from build123d import *

# Parameters (mm, degrees)
CROQUIS1_W              = 195
CROQUIS1_H              = 50
SALIENTE_EXTRUIR1_DEPTH = 4
CROQUIS2_W              = 165
CROQUIS2_H              = 50
SALIENTE_EXTRUIR2_DEPTH = 111
CROQUIS3_W              = 90.257394992
CROQUIS3_H              = 11.130396244
CORTAR_EXTRUIR1_DEPTH   = 10


with BuildPart() as part:
    # Croquis1 → Saliente-Extruir1 (new body)
    with BuildSketch(Plane.XY):
        with Locations((97.5, -25)):
            Rectangle(CROQUIS1_W, CROQUIS1_H)
    extrude(amount=SALIENTE_EXTRUIR1_DEPTH)

    # Croquis2 → Saliente-Extruir2 (add)
    with BuildSketch(Plane(origin=(0, 0, 0), x_dir=(-1, 0, 0), z_dir=(0, 0, -1))):
        with Locations((-97.5, -25)):
            Rectangle(CROQUIS2_W, CROQUIS2_H)
    extrude(amount=SALIENTE_EXTRUIR2_DEPTH)

    # Croquis3 → Cortar-Extruir1 (cut)
    with BuildSketch(Plane(origin=(0, 0, -111), x_dir=(-1, 0, 0), z_dir=(0, 0, -1))):
        with Locations((-97.5, -25)):
            Rectangle(CROQUIS3_W, CROQUIS3_H)
    extrude(amount=-CORTAR_EXTRUIR1_DEPTH, mode=Mode.SUBTRACT)


solid = part.part
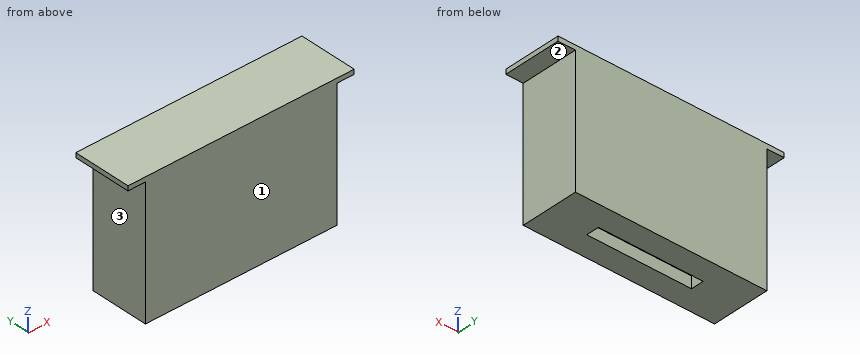
Source: CAD feature listing. Evaluate the final solid. Frame: model axes, mm. Face numbers are marked on the shaded views. A direction names the side the tool comes from. Round coordinates to 2 decimals unless told otherwise and drop trailing zeros. Loops run counter-clockwise (first coordinate to the right, second up) from the corner with the lowest first, then second, coordinate; pieces in that order, holes last. Notation, with made-up numbers: M -9.75,18 L 18.25,18 A7 ccw 18.25,30 Z; hole C -18.75,44.25 d10. An arc over 180 degrees is marked long. Answer as CSV lines item,"result".
Q1. Cut plane B-B (y = -9.5). Return the cut outline in (x, z).
Verdict:
outline,"M 0,0 L 15,0 L 15,-111 L 180,-111 L 180,0 L 195,0 L 195,4 L 0,4 Z"
Q2. Contact query for flat-ended pins moving along their axis: pin 1 (16.5 mm diameter, centred on x = 6.5, y = -28, fed in from -Z); pin 2 (15 mm diameter, centred on y = -21, z = -37, fed in from +X); pin 3 (1 mm diameter, centred on x = 78, y = -24, fed in from -Z). Output: stop coordinate, or through.
Verdict:
pin 1,"stops at z = 0"
pin 2,"stops at x = 180"
pin 3,"stops at z = -101"
Q3. Reachability of the marked faces 1, 2 and 3 from +Z, -Z, +X, -X, +Y, -Y: full face, straight path, thin tool, end or side. Return the list, or none.
Verdict:
face 1,"+Z, -Z, +X, -X, -Y"
face 2,"-Z, +X, +Y, -Y"
face 3,"-Z, -X, +Y, -Y"
Q4. Cut plane A-A (x = 96). Return the cut outline in (y, z).
Verdict:
outline,"M -50,-111 L -30.57,-111 L -30.57,-101 L -19.43,-101 L -19.43,-111 L 0,-111 L 0,4 L -50,4 Z"
Q5. Line query: line 1 along X through (y, z) = (-11, -46); line 2 along Z through (x, y) = (130.5, -25). Output: solid intervals per line, ascending.
Verdict:
line 1,"x = 15 to 180"
line 2,"z = -101 to 4"
Q6. Cut plane C-C (z = -88.5). Return the cut outline in (x, y), plus the area to 3 significant figures.
Verdict:
outline,"M 15,-50 L 180,-50 L 180,0 L 15,0 Z"
area,"8,250 mm^2"
